from build123d import *

# Parameters (mm, degrees)
SKETCH1_R           = 1.5
BOSS_EXTRUDE1_DEPTH = 4


with BuildPart() as part:
    # Sketch1 → Boss-Extrude1 (new body)
    with BuildSketch(Plane.XY):
        with BuildLine():
            Line((0, 0), (0, -96))
            Line((0, -96), (67, -96))
            Line((67, -96), (67, -103))
            ThreePointArc((67, -103), (77, -113), (87, -103))
            Line((87, -103), (87, -96))
            Line((87, -96), (149, -96))
            Line((149, -96), (149, 0))
            Line((149, 0), (87, 0))
            Line((87, 0), (87, 7))
            ThreePointArc((87, 7), (77, 17), (67, 7))
            Line((67, 7), (67, 0))
            Line((67, 0), (0, 0))
        make_face()
        with Locations((77, -103)):
            Circle(SKETCH1_R, mode=Mode.SUBTRACT)
        with Locations((77, 7)):
            Circle(SKETCH1_R, mode=Mode.SUBTRACT)
    extrude(amount=BOSS_EXTRUDE1_DEPTH)


solid = part.part
Could you check a few things on this model? Use its own coordinates, in mm. A direction names the side the tool comes from. Coordinates: 2 decimals unless noted, no trailing zeros. Order: outer loops, then holes, each group sorted by start corner. A loop starts at its lowest first (then second) coordinate and runs counter-clockwise, first axis right, second up.
Q1. Please list where these lines run through material, in increasing order: L1, parallel to Y at x = 77, z = 1.5; L2, parallel to Y at x = 138, z = 2.8; L3, parallel to Y at x = 73.5, z = 0.3.
Q2. Which directions (+Z, -Z, +X, -X, +Y, -Y) give clear straight access to the entire face, cutting with the end or side of a thin tool? Please do faces 1 (the flat face through (118, 0, 2)), 2 (the flat face through (118, -96, 2)), 3 (the flat face through (34, 0, 2)), 4 (the flat face through (33, -96, 2)).
Q3. Suppose I cut it at A-A on z = 2.5. Please give me the cut outline in (x, y), and give its area (3 significant figures).
Q4. Thinking about a two-plate mould opening in X: for faces 5 (the flat face through (87, 3, 2)), 6 (the cylindrical face through (77, 17, 2)), 7 (the cylindrical face through (77.806, -101.735, 1.972)), which applies, released by +X, released by -X, zero draft, split by the parting line, or undercut?
Q5. Suppose I cut it at B-B on x = 47. Please give me the cut outline in (y, z), and give its area (3 significant figures).
Q6. Will these pins go through, and if not, where does the flat tip stop? pin 1 (1.8 mm diameter, centred on x = 77, y = -103, fed in from +Z); pin 2 (1.2 mm diameter, centred on y = 2.5, z = 2, fed in from +X); pin 3 (2 mm diameter, centred on x = 29, z = 1, fed in from -Y); pin 4 (2 mm diameter, centred on x = 111, z = 0.5, fed in from +Y).
Answer:
1. L1: y = -113 to -104.5, -101.5 to 5.5, 8.5 to 17
1. L2: y = -96 to 0
1. L3: y = -112.37 to 16.37
2. face 1: +Z, -Z, +X, +Y
2. face 2: +Z, -Z, +X, -Y
2. face 3: +Z, -Z, -X, +Y
2. face 4: +Z, -Z, -X, -Y
3. outline: (0, -96) - (67, -96) - (67, -103) arc R10 ccw to (87, -103) - (87, -96) - (149, -96) - (149, 0) - (87, 0) - (87, 7) arc R10 ccw to (67, 7) - (67, 0) - (0, 0) - close; hole circle Ø3 at (77, -103); hole circle Ø3 at (77, 7)
3. area: 14,900 mm2
4. face 5: released by +X
4. face 6: split by the parting line
4. face 7: undercut
5. outline: (-96, 0) - (0, 0) - (0, 4) - (-96, 4) - close
5. area: 384 mm2
6. pin 1: passes through
6. pin 2: stops at x = 87
6. pin 3: stops at y = -96
6. pin 4: stops at y = 0
